For this review, use the dimensioned drawing (mm, ordinates from the lowest corner) and the shaded views. A direction names the side the tool comes from. Give positions to 0.01 mm unless a question says otherwise; leave off trailing zeros. Write each loop counter-clockwise with the first axis right and the second up, starting at its lowest first coordinate (ties: lowest second). Pieces come first, ordered by that corner, then holes. Notation, with made-up numbers: M 26,80.5 L 39,80.5 A17 cw 39,112.5 Z; hole C 44,54 d7. An arc over 180 degrees is marked long. Answer in a Markdown table with one row per item.
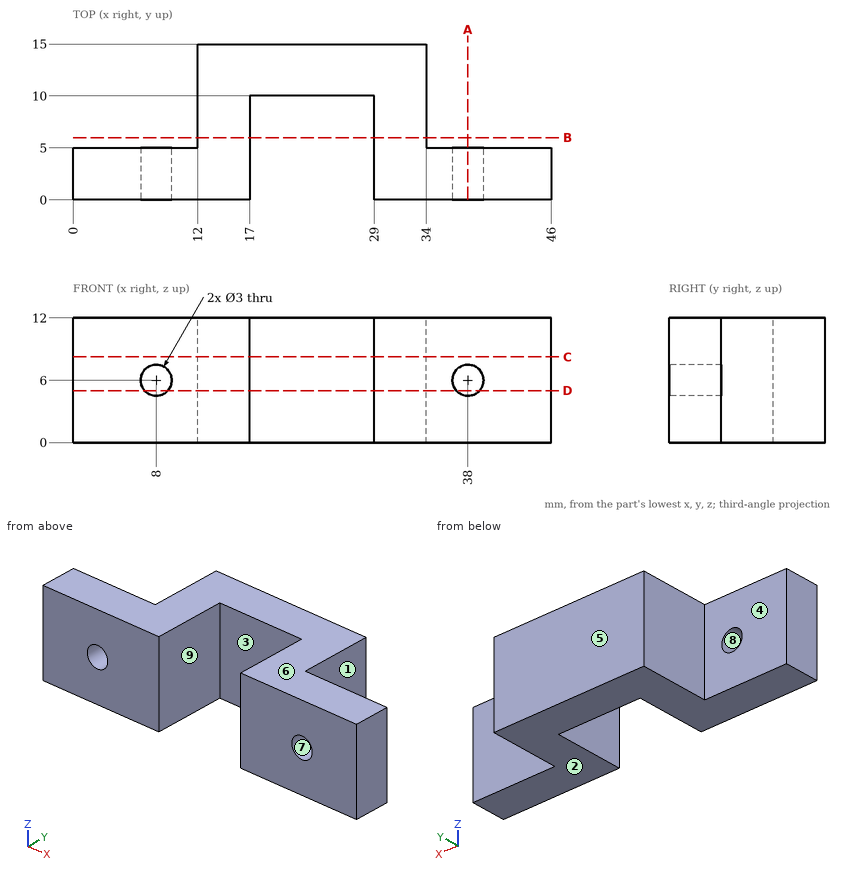
1) The part is to be moulded in two halves that separate along Z. For the marked faces 6, 7, 8 and 9, say which applies: released by +Z, released by -Z, zero draft, split by the parting line, or undercut.
Geometry says:
| item | result |
|---|---|
| face 6 | released by +Z |
| face 7 | undercut |
| face 8 | undercut |
| face 9 | zero draft |
2) To check wall thickness, follow probe 1 along X at (y, z) = (1.15, 6); probe 2 along X at (y, z) = (0.5, 3.5); probe 3 along X at (y, z) = (7.25, 1.25). State the ranges of each line that lie inside material, in increasing order. Write a range as [from, to].
Geometry says:
| item | result |
|---|---|
| probe 1 | [0, 6.5], [9.5, 17], [29, 36.5], [39.5, 46] |
| probe 2 | [0, 17], [29, 46] |
| probe 3 | [12, 17], [29, 34] |
3) Insertion check: P1, Ø4, axis at x = 38, z = 6, coming from the +Y side; P2, Ø1.5, axis at x = 18.5, z = 6.5, coming from the -Y side. Each pin has a flat end and moves straight along its axis. Give the tip position at first contact, or say it passes through.
Geometry says:
| item | result |
|---|---|
| P1 | y = 5 |
| P2 | y = 10 |
4) Add section C-C (z = 8.25). Write out the cut boundary in (x, y).
Geometry says:
| item | result |
|---|---|
| outline | M 0,0 L 17,0 L 17,10 L 29,10 L 29,0 L 46,0 L 46,5 L 34,5 L 34,15 L 12,15 L 12,5 L 0,5 Z |
5) Add section B-B (y = 6). Write out the cut boundary in (x, z).
Geometry says:
| item | result |
|---|---|
| outline | M 12,0 L 17,0 L 17,12 L 12,12 Z; M 29,0 L 34,0 L 34,12 L 29,12 Z |
6) For the marked faces 1, 2, 3, 4 and 5, list the 3-axis set-ups (+Z, -Z, +X, -X, +Y, -Y) from which the entire face can be reached by the end or side of a thin tool; tool diameter is ignored.
Geometry says:
| item | result |
|---|---|
| face 1 | +Z, -Z, +X, +Y |
| face 2 | -Z, +X, -X, +Y, -Y |
| face 3 | +Z, -Z, -Y |
| face 4 | +Z, -Z, -X, +Y |
| face 5 | +Z, -Z, +X, -X, +Y |
7) Add section D-D (z = 5). Write out the cut boundary in (x, y), and give its area (3 significant figures).
Geometry says:
| item | result |
|---|---|
| outline | M 0,0 L 6.88,0 L 6.88,5 L 0,5 Z; M 9.12,0 L 17,0 L 17,10 L 29,10 L 29,0 L 36.88,0 L 36.88,5 L 34,5 L 34,15 L 12,15 L 12,5 L 9.12,5 Z; M 39.12,0 L 46,0 L 46,5 L 39.12,5 Z |
| area | 308 mm^2 |
8) Add section A-A (x = 38). Write out the cut boundary in (y, z), and give its area (3 significant figures).
Geometry says:
| item | result |
|---|---|
| outline | M 0,0 L 5,0 L 5,4.5 L 0,4.5 Z; M 0,7.5 L 5,7.5 L 5,12 L 0,12 Z |
| area | 45.0 mm^2 |
